CAD build for the part. Positions are in the model's coordinates, mm. A direction names the side the tool comes from. Coordinates: 2 decimals unless noted, no trailing zeros. Order: outer loops, then holes, each group sorted by start corner. A loop starts at its lowest first (then second) coordinate and runs counter-clockwise, first axis right, second up. Notation, with made-up numbers: M 85.25,-35 L 97.25,-35 A10 ccw 97.25,-29 Z; hole C 73,-38 d1. An arc over 180 degrees is marked long. Write item = value, one per line. Start each with the question number.
Autodesk Inventor part; units mm, degrees
ref_plane "YZ Plane" through (0, 0, 0) normal (1, 0, 0) x (0, 1, 0)
ref_plane "XZ Plane" through (0, 0, 0) normal (0, 1, 0) x (-1, 0, 0)
ref_plane "XY Plane" through (0, 0, 0) normal (0, 0, 1) x (1, 0, 0)
sketch "Sketch1" plane through (0, 0, 0) normal (0, 0, 1) x (1, 0, 0)
  line L0 (0, 0) -> (0, 10)
  line L1 (0, 0) -> (5, 0)
  line L2 (5, 0) -> (5, 15)
  line L3 (5, 15) -> (4, 15)
  line L4 (4, 15) -> (0, 10)
  dimension "d0" = 10
  dimension "d1" = 5
  dimension "d2" = 15
  dimension "d7" = 1
revolve "Revolution1" add sketch "Sketch1" angle 360 about axis through (0, 0, 0) along (1, 0, 0)
mirror "Mirror1" about plane through (0, 0, 0) normal (1, 0, 0)
sketch "Sketch2" plane through (5, 0, 0) normal (1, 0, 0) x (0, 0, -1)
  circle A0 centre (0, 0) radius 3.1
  dimension "d4" = 6.2
extrude "Extrusion1" cut sketch "Sketch2" against normal through all
sketch "Sketch3" plane through (5, 0, 0) normal (1, 0, 0) x (0, 0, -1)
  point P0 (0, 0)
properties part number "pulley"
1. Slice it at A-A (y = 0). Write the cut outline in (x, z), plus the area to 3 significant figures.
2. 3-axis set-ups, long thin cutter, end or side, ignore diameter. For faces 1 (the cylindrical face through (-4.493, -14.985, 0.66)), 2 (the conical face through (-0.25, -2.236, 10.068)): which of +Z, -Z, +X, -X, +Y, -Y reach the whole face in a straight line?
3. Slice it at D-D (x = 3.25). Write the cut outline in (y, z) (1 decimal), plus the area to 3 significant figures.
4. Slice it at C-C (x = 1). Write the cut outline in (y, z), plus the area to 3 significant figures.
5. Mould opens along Z. For faces 3 (the cylindrical face through (0.07, -2.75, -1.43)), 4 (the flat face through (5, 0, 4)), 5 (the conical face through (0.25, -2.236, -10.068)) say: released by +Z, released by -Z, zero draft, split by the parting line, or undercut.
6. Flat gauge pins, fed straight in: pin 1 (1 mm diameter, centred on x = 0.5, y = 6, fed in from +Z); pin 2 (2 mm diameter, centred on x = 0.5, y = 9, fed in from -Z); pin 3 (5 mm diameter, centred on y = 0, z = 0, fed in from -X); pin 4 (3 mm diameter, centred on x = 0.5, y = -5.5, fed in from +Z). Where does each tip first touch, or does it go through?
7. Probe L1, parallel to X at y = 10.5, z = -1; L2, parallel to X at y = 8.75, z = 7.5; L3, parallel to Y at x = 2.25, z = 0. List the from-to ranges inside material, lowest first.
Calculated:
q1.outline = M -5,-15 L -4,-15 L 0,-10 L 4,-15 L 5,-15 L 5,-3.1 L -5,-3.1 Z; M -5,3.1 L 5,3.1 L 5,15 L 4,15 L 0,10 L -4,15 L -5,15 Z
q1.area = 198 mm²
q2.face_1 = +X, -X
q2.face_2 = none
q3.outline = C 0,0 d28.1; hole C 0,0 d6.2
q3.area = 591 mm²
q4.outline = C 0,0 d22.5; hole C 0,0 d6.2
q4.area = 367 mm²
q5.face_3 = undercut
q5.face_4 = zero draft
q5.face_5 = split by the parting line
q6.pin_1 = 9.58
q6.pin_2 = -8.05
q6.pin_3 = through
q6.pin_4 = 11.34
q7.L1 = -5 to -0.44, 0.44 to 5
q7.L2 = -5 to -1.22, 1.22 to 5
q7.L3 = -12.81 to -3.1, 3.1 to 12.81
